from build123d import *

# Parameters (mm, degrees)
F0_R     = 3.175
F1_DEPTH = 304.8


with BuildPart() as f1:
    # F0 (on Front) → F1 (new body)
    with BuildSketch(Plane.XZ):
        with BuildLine():
            ThreePointArc((-9.525, 114.3), (0, 104.775), (9.525, 114.3))
            ThreePointArc((9.525, 114.3), (0, 123.825), (-9.525, 114.3))
        make_face()
        with Locations((0, 114.3)):
            Circle(F0_R, mode=Mode.SUBTRACT)
        with BuildLine():
            Line((15.386538, 67.407692), (9.525, 114.3))
            ThreePointArc((9.525, 114.3), (0, 104.775), (-9.525, 114.3))
            Line((-9.525, 114.3), (-15.747457, 65.50829))
            ThreePointArc((-15.747457, 65.50829), (-0.966694, 79.34554), (15.386538, 67.407692))
        make_face()
        with Locations((-3.175, 100.0252)):
            Circle(F0_R, mode=Mode.SUBTRACT)
        with BuildLine():
            Line((15.875, 63.5), (15.386538, 67.407692))
            ThreePointArc((15.386538, 67.407692), (-0.966694, 79.34554), (-15.747457, 65.50829))
            ThreePointArc((-15.747457, 65.50829), (-15.873588, 63.711757), (-15.795426, 61.9125))
            ThreePointArc((-15.795426, 61.9125), (0, 47.625), (15.795426, 61.9125))
            ThreePointArc((15.795426, 61.9125), (15.855094, 62.705253), (15.875, 63.5))
        make_face()
        with Locations((0, 63.5)):
            Circle(F0_R, mode=Mode.SUBTRACT)
        with BuildLine():
            ThreePointArc((15.875, 63.5), (15.752411, 65.469051), (15.386538, 67.407692))
            Line((15.386538, 67.407692), (15.875, 63.5))
        make_face()
        with BuildLine():
            ThreePointArc((15.795426, 61.9125), (0, 47.625), (-15.795426, 61.9125))
            Line((-15.795426, 61.9125), (-9.477255, -0.9525))
            ThreePointArc((-9.477255, -0.9525), (-0.476848, 9.513056), (9.525, 0))
            ThreePointArc((9.525, 0), (6.854408, -6.613827), (0.340179, -9.518923))
            Line((0.340179, -9.518923), (44.733482, -7.932436))
            ThreePointArc((44.733482, -7.932436), (36.5125, 0), (44.733482, 7.932436))
            Line((44.733482, 7.932436), (18.9676, 8.853234))
            ThreePointArc((18.9676, 8.853234), (13.2612, 11.571359), (11.341187, 17.593382))
            Line((11.341187, 17.593382), (15.795426, 61.9125))
        make_face()
        with BuildLine():
            ThreePointArc((9.525, 0), (-0.476848, 9.513056), (-9.477255, -0.9525))
            ThreePointArc((-9.477255, -0.9525), (-6.262383, -7.17692), (0.340179, -9.518923))
            ThreePointArc((0.340179, -9.518923), (6.854408, -6.613827), (9.525, 0))
        make_face()
        Circle(F0_R, mode=Mode.SUBTRACT)
        with BuildLine():
            ThreePointArc((44.733482, 7.932436), (36.5125, 0), (44.733482, -7.932436))
            ThreePointArc((44.733482, -7.932436), (50.162007, -5.511523), (52.3875, 0))
            ThreePointArc((52.3875, 0), (50.162007, 5.511523), (44.733482, 7.932436))
        make_face()
        with Locations((44.45, 0)):
            Circle(F0_R, mode=Mode.SUBTRACT)
    extrude(amount=F1_DEPTH)


solid = f1.part
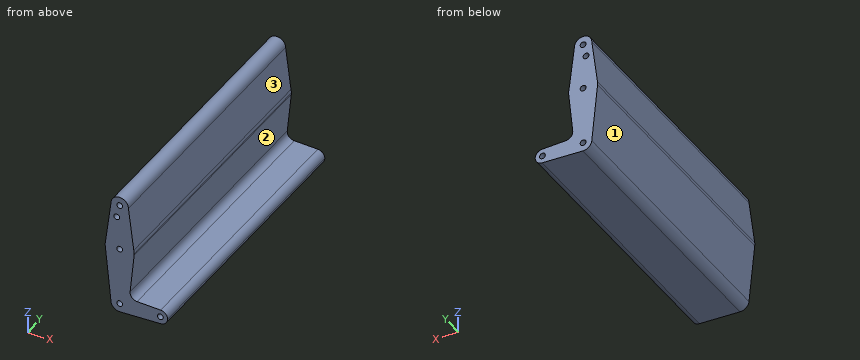
Verification items for the finished model (mm, model axes). Face numbers are marked on the shaded views. Coordinates: 2 decimals unless noted, no trailing zeros. Loops run counter-clockwise (first coordinate to the right, second up) from the corner with the lowest first, then second, coordinate; pieces in that order, holes last. Notation, with made-up numbers: (-36, 62.25) -> (1, 62.25) arc R25 cw to (1, 97.25) -> close; hole circle Ø1 at (48.25, 68). An arc over 180 degrees is marked (long way). Answer as a JSON object with one key per item and string values. Group by question number.
Item 1: Mould release check, pull along Z, two halves, no side actions. Record for the marked faces 1, 2 and 3: +Z half, -Z half, draft (parallel to the pull), parting line (faces both ways), or undercut.
Item 2: Depth check by flat-ended pin: pin 1 (10 mm diameter, centred on x = 6, y = -34, fed in from +Z); pin 2 (6 mm diameter, centred on x = 36, y = -241, fed in from +Z); pin 3 (10 mm diameter, centred on x = 44, y = -50, fed in from -Z). Enter the tip coordinate at first touch or a pass-through.
Item 3: Scan lines: probe 1 along X at (y, z) = (-113, 114); probe 2 along Z at (x, y) = (44.5, -129.5); probe 3 along X at (y, z) = (-179.5, -1). Record each from-to range of solid material in increasing order.
Item 4: Sectioned sample at A-A on y = -267.5. State how many separate pieces and enclosed holes the cut face has, plus the area to 3 significant figures.
Item 5: Sectioned sample at B-B on x = 6. Record the boundary of the cut face in (y, z), plus the area to 3 significant figures.
Evaluation:
{
 "1": {"face 1": "-Z half", "face 2": "undercut", "face 3": "+Z half"},
 "2": {"pin 1": "stops at z = 123.77", "pin 2": "stops at z = 8.35", "pin 3": "stops at z = -8.14"},
 "3": {"probe 1": "x = -9.56 to -3.16, 3.16 to 9.56", "probe 2": "z = -7.94 to -3.17, 3.17 to 7.94", "probe 3": "x = -9.47 to -3.01, 3.01 to 41.44, 47.46 to 52.32"},
 "4": {"separate pieces": "1", "enclosed holes": "5", "area": "3,770 mm²"},
 "5": {"outline": "(-304.8, -9.32) -> (0, -9.32) -> (0, 121.7) -> (-304.8, 121.7) -> close", "area": "39,900 mm²"}
}
